```python
from build123d import *

# Parameters (mm, degrees)
EXTRUDE_1_DEPTH     = 40
EXTRUDE_2_DEPTH     = 40
CUT_EXTRUDE_1_DEPTH = 40
CUT_EXTRUDE_2_DEPTH = 40


with BuildPart() as part:
    # 草图1 → 凸台-拉伸1 (new body)
    with BuildSketch(Plane(origin=(0, 0, 0), x_dir=(1, 0, 0), z_dir=(0, 1, 0))):
        Polygon((-6.780821918, 7.191780822), (13.219178082, 7.191780822), (13.219178082, -32.808219178), (-6.780821918, -32.808219178), (-26.780821918, -32.808219178), (-26.780821918, -12.808219178), (-6.780821918, -12.808219178), align=None)
    extrude(amount=EXTRUDE_1_DEPTH)

    # 草图2 → 凸台-拉伸2 (add)
    with BuildSketch(Plane.XZ):
        Polygon((-6.780821918, -7.191780822), (-26.780821918, 12.808219178), (-6.780821918, 12.808219178), align=None)
    extrude(amount=-EXTRUDE_2_DEPTH)

    # 草图3 → 切除-拉伸1 (cut)
    with BuildSketch(Plane.XY.offset(12.808219178)):
        Polygon((-6.780821918, 40), (-26.780821918, 0), (-26.780821918, 40), align=None)
    extrude(amount=-CUT_EXTRUDE_1_DEPTH, mode=Mode.SUBTRACT)

    # 草图4 → 切除-拉伸2 (cut)
    with BuildSketch(Plane(origin=(-6.780821918, 0, 0), x_dir=(0, 0, -1), z_dir=(1, 0, 0))):
        Polygon((-12.808219178, 40), (7.191780822, 0), (7.191780822, 40), align=None)
    extrude(amount=-CUT_EXTRUDE_2_DEPTH, mode=Mode.SUBTRACT)


solid = part.part
```
Can you work these out from the model? Positions are in its coordinate system, mm. A direction names the side the tool comes from. Give positions to 0.01 mm unless a question says otherwise; leave off trailing zeros. Loops run counter-clockwise (first coordinate to the right, second up) from the corner with the lowest first, then second, coordinate; pieces in that order, holes last. Notation, with made-up numbers: M -9,35 L 32,35 A21 cw 32,50 Z; hole C -32,-35 d3. An arc over 180 degrees is marked long. Use one line per item in the form item = value. Start each with the question number.
(1) Please list where these lines run through material, in increasing order: line 1 (X direction, y = 23, z = -2.5); line 2 (Z direction, x = -20, y = 17.5); line 3 (Z direction, x = -10.5, y = 29.5).
(2) On a 3-axis mill with a long thin cutter (end or side, diameter ignored), from which of +Z, -Z, +X, -X, +Y, -Y can I reach the whole of each face in a straight line? I mean faces 4 (the flat face through (-16.64, 20.28, 8.99)), 5 (the flat face through (3, 20, -7.192)). Say none if no direction works.
(3) Thinking about a two-plate mould opening in Y: for faces 1 (the flat face through (-16.64, 7.64, 2.67)), 2 (the flat face through (-7, 0, 13)), 3 (the flat face through (-2, 40, 18)), which applies, released by +Y, released by -Y, zero draft, split by the parting line, or undercut?
(4) I want a section at C-C, the plane x = -8.5. Write out the boundary of the cut face in (y, z), and give its area (3 significant figures).
(5) I'm going to push a flat-ended pin straight in: P1, Ø6, axis at y = 13, z = 4.5, coming from the -X side. Where does the tip first touch, or does it pass through?
(6) I want a section at B-B, the plane y = 37.5. Write out the boundary of the cut face in (x, z).
(7) I want a section at A-A, the plane z = 4. Write out the boundary of the cut face in (x, y), and give its area (3 significant figures).
(8) I want a section at D-D, the plane x = -21.5. Write out the boundary of the cut face in (y, z), and give its area (3 significant figures).
Worked out:
q1.line_1 = -6.78 to 13.22
q1.line_2 = 12.81 to 32.81
q1.line_3 = 7.56 to 32.81
q2.face_4 = -Z, -X, +Y
q2.face_5 = -Z, +X, -X, +Y, -Y
q3.face_1 = zero draft
q3.face_2 = released by -Y
q3.face_3 = released by +Y
q4.outline = M 0,-5.47 L 3.44,-5.47 L 36.56,11.09 L 36.56,12.81 L 40,12.81 L 40,32.81 L 0,32.81 Z
q4.area = 1,190 mm²
q5.P1 = -21.05
q6.outline = M -26.78,12.81 L -8.03,12.81 L -8.03,11.56 L -6.78,11.56 L -6.78,-7.19 L 13.22,-7.19 L 13.22,32.81 L -26.78,32.81 Z
q7.outline = M -17.97,0 L 13.22,0 L 13.22,40 L -6.78,40 L -6.78,22.38 L -15.59,22.38 L -17.97,17.62 Z
q7.area = 1,040 mm²
q8.outline = M 0,7.53 L 10.56,7.53 L 10.56,12.81 L 40,12.81 L 40,32.81 L 0,32.81 Z
q8.area = 856 mm²
